Could you check a few things on this model? Use its own coordinates, in mm. A direction names the side the tool comes from. Give positions to 0.01 mm unless a question says otherwise; leave off trailing zeros. Loops run counter-clockwise (first coordinate to the right, second up) from the corner with the lowest first, then second, coordinate; pieces in that order, holes last.
1. Imagine slicing it at C-C (y = 15). List the corners of the cut face in (x, z) for me, plus the area to 3 significant figures.
2. I need wall thicknesses on line 1 along Z through (x, y) = (-5, -19.5); line 2 along Z through (x, y) = (12, -29.5); line 3 along Y through (x, z) = (13, -1). Which ranges of each line are inside material? Lowest first, please.
3. Imagine slicing it at D-D (x = 8). List the corners of the cut face in (y, z) for me, plus the area to 3 significant figures.
4. Thinking about a two-plate mould opening in Y: for faces 1 (the flat face through (18, -44, 0)), 2 (the flat face through (25, -35, -17)), 3 (the flat face through (35, -45, 0)), 4 (the cylindrical face through (-23.09, 9.58, 0.63)), which applies, +Y half, -Y half, draft (parallel to the pull), parting line (faces both ways), or undercut?
5. Imagine slicing it at A-A (z = -5). List the corners of the cut face in (x, y) for me.
6. For P1, Ø6, axis at x = 6, y = 19.5, coming from the -Z side; P2, Ø12, axis at x = 2, y = -28.5, coming from the +Z side; P3, Ø1, axis at y = -36.5, z = 20, coming from the -X side; P4, Ø3, axis at y = 14, z = -10.5, coming from the +X side, each with a flat end and sliding along its axis, tell me the tip position at first contact or that it passes through.
7. Imagine slicing it at B-B (x = -20). List the corners of the cut face in (y, z) for me, plus the area to 3 significant figures.
8. For faces 5 (the flat face through (0, -47, 0)), 6 (the flat face through (5, -22, 9)), 7 (the flat face through (0, 13, -40)), 8 (the flat face through (0, 13, 40)), which set-ups out of +Z, -Z, +X, -X, +Y, -Y let a thin tool reach every point of the face, with its end or its side?
```python
from build123d import *

# Parameters (mm, degrees)
CROQUIS1_R                 = 25
SALIENTE_EXTRUIR1_DEPTH    = 45
CORTAR_EXTRUIR1_DEPTH      = 10
CORTAR_EXTRUIR2_START      = -80
CORTAR_EXTRUIR2_DEPTH      = 10
CROQUIS3_W                 = 35
CROQUIS3_H                 = 50
SALIENTE_EXTRUIR2_DEPTH    = 68
CORTAR_EXTRUIR4_DEPTH      = 89.735562206
CORTAR_EXTRUIR4_DEPTH_BACK = 48
CROQUIS4_W                 = 20
CROQUIS4_H                 = 50
CROQUIS5_W                 = 18
CROQUIS5_H                 = 45
CORTAR_EXTRUIR5_DEPTH      = 94.005376189


with BuildPart() as part:
    # Croquis1 → Saliente-Extruir1 (new, symmetric)
    with BuildSketch(Plane.XY):
        with Locations(Location((0, 0, 0), (0, 0, 180))):
            Circle(CROQUIS1_R)
    extrude(amount=SALIENTE_EXTRUIR1_DEPTH, both=True)

    # Croquis2 → Cortar-Extruir1 (cut)
    with BuildSketch(Plane.XY.offset(45)):
        with BuildLine():
            Line((-21.354156504, 13), (21.354156504, 13))
            ThreePointArc((21.354156504, 13), (0, 25), (-21.354156504, 13))
        make_face()
    extrude(amount=-CORTAR_EXTRUIR1_DEPTH, mode=Mode.SUBTRACT)

    # Croquis2<2> → Cortar-Extruir2 (cut)
    with BuildSketch(Plane.XY.offset(45).offset(CORTAR_EXTRUIR2_START)):
        with BuildLine():
            Line((-21.354156504, 13), (21.354156504, 13))
            ThreePointArc((21.354156504, 13), (0, 25), (-21.354156504, 13))
        make_face()
    extrude(amount=-CORTAR_EXTRUIR2_DEPTH, mode=Mode.SUBTRACT)

    # Croquis3 → Saliente-Extruir2 (add)
    with BuildSketch(Plane(origin=(0, -55, 0), x_dir=(1, 0, 0), z_dir=(0, 1, 0))):
        with Locations((17.5, 0)):
            Rectangle(CROQUIS3_W, CROQUIS3_H)
    extrude(amount=SALIENTE_EXTRUIR2_DEPTH)

    # Croquis4 → Cortar-Extruir4 (cut, two sides: drawn at the far end of the back side and taken through both)
    with BuildSketch(Plane(origin=(0, 13, 0), x_dir=(1, 0, 0), z_dir=(0, 1, 0)).offset(-CORTAR_EXTRUIR4_DEPTH_BACK)):
        with Locations((25, 0)):
            Rectangle(CROQUIS4_W, CROQUIS4_H)
    extrude(amount=CORTAR_EXTRUIR4_DEPTH + CORTAR_EXTRUIR4_DEPTH_BACK, mode=Mode.SUBTRACT)

    # Croquis5 → Cortar-Extruir5 (cut, through all)
    with BuildSketch(Plane(origin=(35, 0, 0), x_dir=(0, 0, -1), z_dir=(1, 0, 0))):
        with Locations((0, -21.5)):
            Rectangle(CROQUIS5_W, CROQUIS5_H)
    extrude(amount=-CORTAR_EXTRUIR5_DEPTH, mode=Mode.SUBTRACT)


solid = part.part
```
Derived:
1. outline: (-20, -35) - (20, -35) - (20, -25) - (15, -25) - (15, 25) - (20, 25) - (20, 35) - (-20, 35) - close
1. area: 2,550 mm2
2. line 1: z = -45 to -9, 9 to 45
2. line 2: z = -25 to -9, 9 to 25
2. line 3: y = -55 to -44, 1 to 21.35
3. outline: (-55, -25) - (-23.69, -25) - (-23.69, -45) - (13, -45) - (13, -35) - (23.69, -35) - (23.69, 35) - (13, 35) - (13, 45) - (-23.69, 45) - (-23.69, 25) - (-55, 25) - close; hole (-44, -9) - (1, -9) - (1, 9) - (-44, 9) - close
3. area: 4,810 mm2
4. face 1: undercut
4. face 2: +Y half
4. face 3: draft
4. face 4: parting line
5. outline: (-24.98, 1) - (15, 1) - (15, 20) arc R25 ccw to start; (0, -55) - (35, -55) - (35, -44) - (0, -44) - close
6. P1: stops at z = -35
6. P2: stops at z = 45
6. P3: stops at x = 0
6. P4: stops at x = 15
7. outline: (-15, -45) - (13, -45) - (13, -35) - (15, -35) - (15, 35) - (13, 35) - (13, 45) - (-15, 45) - (-15, 9) - (1, 9) - (1, -9) - (-15, -9) - close
7. area: 2,370 mm2
8. face 5: +Z, -Z, -X, -Y
8. face 6: +X, -X
8. face 7: -Z, +X, -X, +Y
8. face 8: +Z, +X, -X, +Y
